from build123d import *

# Parameters (mm, degrees)
BOSS_EXTRUDE1_DEPTH = 5
BOSS_EXTRUDE3_DEPTH = 20
SKETCH5_W           = 9
SKETCH5_H           = 18
CUT_EXTRUDE3_DEPTH  = 20
SKETCH6_R           = 3.5
SKETCH6_R_2         = 1.5
BOSS_EXTRUDE4_DEPTH = 5
SKETCH7_R           = 2
CUT_EXTRUDE4_DEPTH  = 5


with BuildPart() as part:
    # Sketch1 → Boss-Extrude1 (new body)
    with BuildSketch(Plane(origin=(0, 0, 0), x_dir=(1, 0, 0), z_dir=(0, 1, 0))):
        Polygon((14.142135624, 0), (84.142135624, 0), (91.213203436, -7.071067812), (98.284271247, 0), (105.355339059, 7.071067812), (98.284271247, 14.142135624), (98.284271247, 84.142135624), (105.355339059, 84.142135624), (105.355339059, 104.142135624), (98.284271247, 104.142135624), (98.284271247, 174.142135624), (105.355339059, 181.213203436), (98.284271247, 188.284271247), (91.213203436, 195.355339059), (84.142135624, 188.284271247), (14.142135624, 188.284271247), (7.071067812, 195.355339059), (0, 188.284271247), (-7.071067812, 181.213203436), (0, 174.142135624), (0, 104.142135624), (-7.071067812, 104.142135624), (-7.071067812, 84.142135624), (0, 84.142135624), (0, 14.142135624), (-7.071067812, 7.071067812), (0, 0), (7.071067812, -7.071067812), align=None)
    extrude(amount=BOSS_EXTRUDE1_DEPTH)

    # Sketch4 → Boss-Extrude3 (add)
    with BuildSketch(Plane(origin=(0, 5, 0), x_dir=(1, 0, 0), z_dir=(0, 1, 0))):
        Polygon((0, 174.142135624), (14.142135624, 188.284271247), (84.142135624, 188.284271247), (98.284271247, 174.142135624), (98.284271247, 14.142135624), (84.142135624, 0), (14.142135624, 0), (0, 14.142135624), align=None)
        Polygon((3, 15.384776311), (3, 172.899494937), (15.384776311, 185.284271247), (82.899494937, 185.284271247), (95.284271247, 172.899494937), (95.284271247, 15.384776311), (82.899494937, 3), (15.384776311, 3), align=None, mode=Mode.SUBTRACT)
    extrude(amount=BOSS_EXTRUDE3_DEPTH)

    # Sketch5 → Cut-Extrude3 (cut)
    with BuildSketch(Plane(origin=(0, 5, 0), x_dir=(1, 0, 0), z_dir=(0, 1, 0))):
        Polygon((70, 15.556349186), (76.363961031, 9.192388155), (82.727922061, 15.556349186), (89.091883092, 21.920310217), (82.727922061, 28.284271247), align=None)
        Polygon((21.920310217, 9.192388155), (15.556349186, 15.556349186), (9.192388155, 21.920310217), (15.556349186, 28.284271247), (28.284271247, 15.556349186), align=None)
        with Locations((13.702828803, 94.142135624)):
            Rectangle(SKETCH5_W, SKETCH5_H)
        with Locations((84.581442444, 94.142135624)):
            Rectangle(SKETCH5_W, SKETCH5_H)
        Polygon((76.363961031, 179.091883092), (82.727922061, 172.727922061), (89.091883092, 166.363961031), (82.727922061, 160), (70, 172.727922061), align=None)
        Polygon((15.556349186, 160), (28.284271247, 172.727922061), (21.920310217, 179.091883092), (15.556349186, 172.727922061), (9.192388155, 166.363961031), align=None)
    extrude(amount=-CUT_EXTRUDE3_DEPTH, mode=Mode.SUBTRACT)

    # Sketch6 → Boss-Extrude4 (add)
    with BuildSketch(Plane(origin=(0, 25, 0), x_dir=(1, 0, 0), z_dir=(0, 1, 0))):
        with Locations((16.907704548, 183.761343011)):
            Circle(SKETCH6_R)
        with Locations((16.907704548, 183.761343011)):
            Circle(SKETCH6_R_2, mode=Mode.SUBTRACT)
        with Locations((81.3765667, 183.761343011)):
            Circle(SKETCH6_R)
        with Locations((81.3765667, 183.761343011)):
            Circle(SKETCH6_R_2, mode=Mode.SUBTRACT)
        with Locations((81.3765667, 4.522928237)):
            Circle(SKETCH6_R)
        with Locations((81.3765667, 4.522928237)):
            Circle(SKETCH6_R_2, mode=Mode.SUBTRACT)
        with Locations((16.907704548, 4.522928237)):
            Circle(SKETCH6_R)
        with Locations((16.907704548, 4.522928237)):
            Circle(SKETCH6_R_2, mode=Mode.SUBTRACT)
    extrude(amount=-BOSS_EXTRUDE4_DEPTH)

    # Sketch7 → Cut-Extrude4 (cut)
    with BuildSketch(Plane(origin=(0, 5, 0), x_dir=(1, 0, 0), z_dir=(0, 1, 0))):
        with Locations((7.778174593, 188.284271247)):
            Circle(SKETCH7_R)
        with Locations((0, 180.506096654)):
            Circle(SKETCH7_R)
        with Locations((90.506096654, 188.284271247)):
            Circle(SKETCH7_R)
        with Locations((98.284271247, 180.506096654)):
            Circle(SKETCH7_R)
        with Locations((99.855339059, 99.642135624)):
            Circle(SKETCH7_R)
        with Locations((99.855339059, 88.642135624)):
            Circle(SKETCH7_R)
        with Locations((98.284271247, 7.778174593)):
            Circle(SKETCH7_R)
        with Locations((90.506096654, 0)):
            Circle(SKETCH7_R)
        with Locations((7.778174593, 0)):
            Circle(SKETCH7_R)
        with Locations((0, 7.778174593)):
            Circle(SKETCH7_R)
        with Locations((-1.571067812, 88.642135624)):
            Circle(SKETCH7_R)
        with Locations((-1.571067812, 99.642135624)):
            Circle(SKETCH7_R)
    extrude(amount=-CUT_EXTRUDE4_DEPTH, mode=Mode.SUBTRACT)


solid = part.part
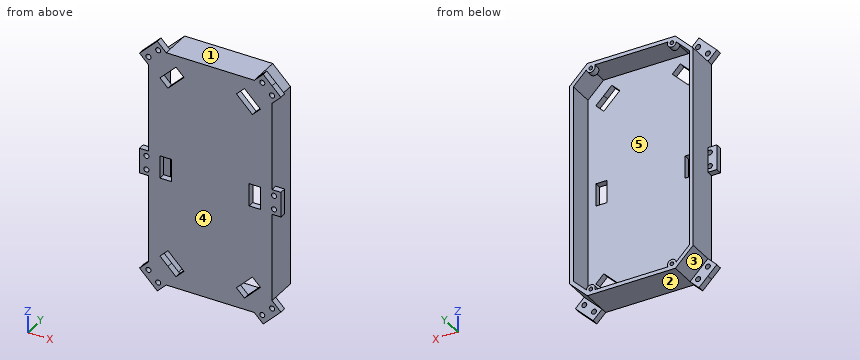
Can you work these out from the model? Positions are in its coordinate system, mm. Face numbers are marked on the shaded views. A direction names the side the tool comes from. Give positions to 0.01 mm unless a question says otherwise; leave off trailing zeros. Loops run counter-clockwise (first coordinate to the right, second up) from the corner with the lowest first, then second, coordinate; pieces in that order, holes last. Notation, with made-up numbers: (62.5, 46) -> (89.5, 46) arc R29 cw to (89.5, 66) -> close; hole circle Ø7 at (-35, 84.25). An arc over 180 degrees is marked (long way). Return JSON: item names as keys, results as strings.
Q1. I need wall thicknesses on probe 1 along X at (y, z) = (23.5, -153); probe 2 along Z at (x, y) = (70.5, 20.75); probe 3 along Z at (x, y) = (58.5, 3.5). Which ranges of each line are inside material? Lowest first, please.
Checks:
{"probe 1": "x = 0 to 3, 95.28 to 98.28", "probe 2": "z = -188.28 to -185.28, -3 to 0", "probe 3": "z = -188.28 to 0"}
Q2. I want a section at C-C, the plane y = 2.25. Count the separate pieces of the cut face and the enclosed holes in it, then the cut area to 3 significant figures.
Checks:
{"separate pieces": "1", "enclosed holes": "18", "area": "18,100 mm2"}
Q3. I want a section at B-B, the plane z = -74. List the corners of the cut face in (x, y) for me.
Checks:
{"outline": "(0, 0) -> (98.28, 0) -> (98.28, 25) -> (95.28, 25) -> (95.28, 5) -> (3, 5) -> (3, 25) -> (0, 25) -> close"}
Q4. We'd pull the mould along Z, two halves only. Please class the marked faces 3, 4 and 5: released by +Z, released by -Z, zero draft, split by the parting line, or undercut.
Checks:
{"face 3": "released by -Z", "face 4": "zero draft", "face 5": "undercut"}
Q5. On a 3-axis mill with a long thin cutter (end or side, diameter ignored), from which of +Z, -Z, +X, -X, +Y, -Y can I reach the whole of each face in a straight line? I mean the marked faces 1 and 2. Say none if no direction works.
Checks:
{"face 1": "+Z, +Y, -Y", "face 2": "-Z, +Y, -Y"}
Q6. For pin 1 Ø5.5 at (x, y) = (13, 2.5) entering from -Z; pin 2 Ø1 at (x, y) = (77, 6) entering from +Z; pin 3 Ø6.5 at (x, z) = (97, -4) entering from +Y; pin 4 Ø2.5 at (x, z) = (90.51, 0) entering from +Y, each with a flat end and sliding along its axis, tell me the tip position at first contact or that it passes through.
Checks:
{"pin 1": "stops at z = -192.18", "pin 2": "stops at z = 0", "pin 3": "stops at y = 5", "pin 4": "passes through"}
Q7. I want a section at A-A, the plane y = 12.5. List the corners of the cut face in (x, z) for me, then the cut area to 3 significant figures.
Checks:
{"outline": "(0, -174.14) -> (14.14, -188.28) -> (84.14, -188.28) -> (98.28, -174.14) -> (98.28, -14.14) -> (84.14, 0) -> (14.14, 0) -> (0, -14.14) -> close; hole (3, -172.9) -> (15.38, -185.28) -> (82.9, -185.28) -> (95.28, -172.9) -> (95.28, -15.38) -> (82.9, -3) -> (15.38, -3) -> (3, -15.38) -> close", "area": "1,590 mm2"}
